Study the drawing (mm; zero at the part's minimum x, y, z) and answer. A direction names the side the tool comes from. Round coordinates to 2 decimals unless told otherwise and drop trailing zeros. Write each loop counter-clockwise with the first axis right and the second up, starting at its lowest first coordinate (ties: lowest second). Pieces come first, ordered by that corner, then holes. Notation, with made-up numbers: M -30,29 L -3,29 A16 cw -3,40 Z; hole C -4,30 d9. An arc over 180 degrees is marked long. Write each question's results on one line, items separated by ' | '.
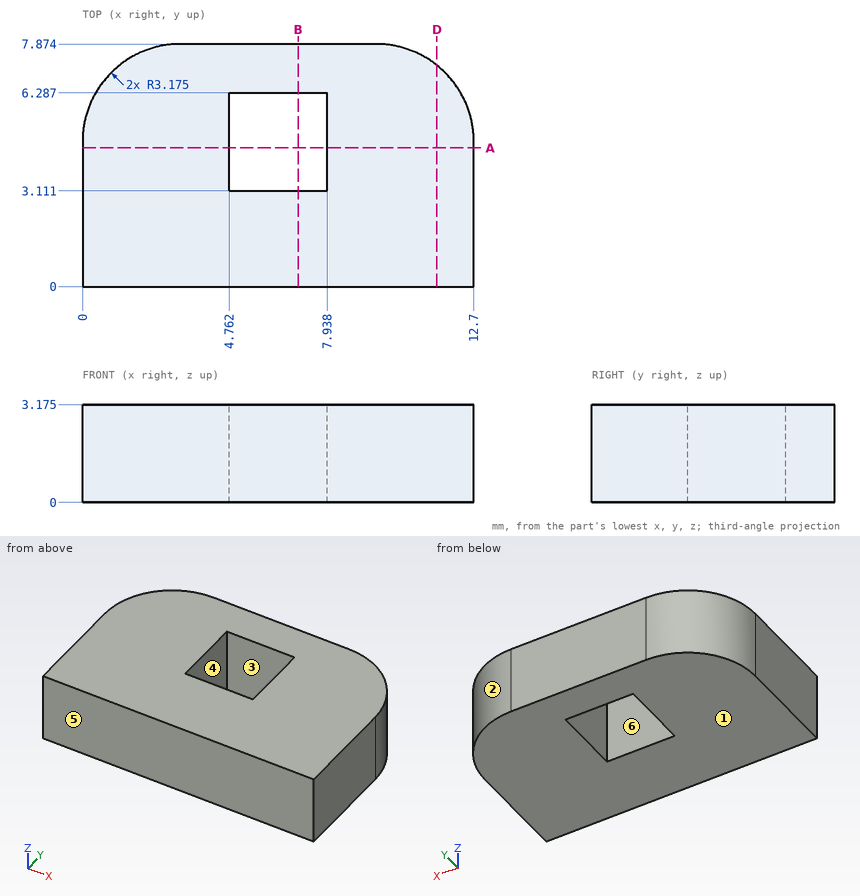
1) The mould has two halves that part along Y. Classify the marked faces 1, 2, 3 and 4: +Y half, -Y half, draft (parallel to the pull), parting line (faces both ways), or undercut.
Return value:
face 1: draft | face 2: +Y half | face 3: undercut | face 4: undercut
2) Find the intervals of material crossed by line 1 (X direction, y = 4.25, z = 1.8); line 2 (Y direction, x = 6.75, z = 2.4) (1 decimal); line 3 (X direction, y = 5.5, z = 2.5), in increasing order.
Return value:
line 1: 0 to 4.76, 7.94 to 12.7 | line 2: 0 to 3.1, 6.3 to 7.9 | line 3: 0.1 to 4.76, 7.94 to 12.6
3) Each of these flat-tipped pins is pushed along its axis until it touches: pin 1 (1 mm diameter, centred on x = 5, y = 6.5, fed in from -Z); pin 2 (1.5 mm diameter, centred on y = 7, z = 0.5, fed in from +X) (1 decimal). Where does it stop, or does it pass through?
Return value:
pin 1: z = 0 | pin 2: x = 12.3
4) Section A-A (y = 4.5) is taken. Determine the outline of the cut face in (x, z) (1 decimal).
Return value:
outline: M 0,0 L 4.8,0 L 4.8,3.2 L 0,3.2 Z; M 7.9,0 L 12.7,0 L 12.7,3.2 L 7.9,3.2 Z
5) Section D-D (x = 11.5) is taken. Determine the outline of the cut face in (y, z) (1 decimal), then the cut area to 3 significant figures.
Return value:
outline: M 0,0 L 7.2,0 L 7.2,3.2 L 0,3.2 Z | area: 22.8 mm²
6) Section B-B (x = 7) is taken. Determine the outline of the cut face in (y, z) (1 decimal).
Return value:
outline: M 0,0 L 3.1,0 L 3.1,3.2 L 0,3.2 Z; M 6.3,0 L 7.9,0 L 7.9,3.2 L 6.3,3.2 Z
7) A tool of negligible diameter and unlimited length cuts with its end or side. For the marked faces 5 and 6, from which of +Z, -Z, +X, -X, +Y, -Y can it reach the whole face along a straight path? Write none if from no direction.
Return value:
face 5: +Z, -Z, +X, -X, -Y | face 6: +Z, -Z
